Could you check a few things on this drawing? It's one solid part, dimensions in mm from its lowest x, y, z. Coordinates: 2 decimals unless noted, no trailing zeros. Order: outer loops, then holes, each group sorted by start corner. A loop starts at its lowest first (then second) coordinate and runs counter-clockwise, first axis right, second up.
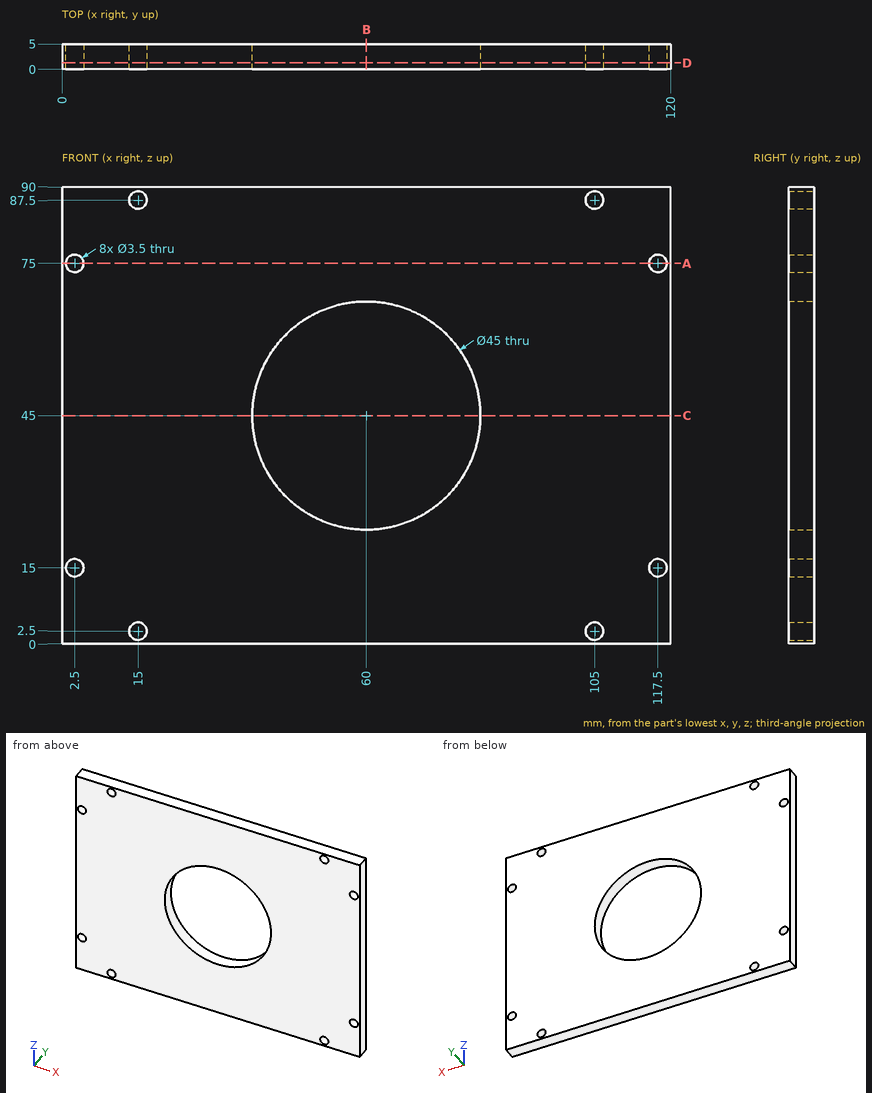
1. Imagine slicing it at A-A on z = 75. Please give me the cut outline in (x, y).
Completed:
outline: (0, 0) - (0.75, 0) - (0.75, 5) - (0, 5) - close; (4.25, 0) - (115.75, 0) - (115.75, 5) - (4.25, 5) - close; (119.25, 0) - (120, 0) - (120, 5) - (119.25, 5) - close
2. Please list where these lines run through material, in increasing order: probe 1 along X at (y, z) = (3.15, 2.5); probe 2 along Z at (x, y) = (105, 3.7); probe 3 along Z at (x, y) = (2.5, 2).
Completed:
probe 1: x = 0 to 13.25, 16.75 to 103.25, 106.75 to 120
probe 2: z = 0 to 0.75, 4.25 to 85.75, 89.25 to 90
probe 3: z = 0 to 13.25, 16.75 to 73.25, 76.75 to 90
3. Imagine slicing it at B-B on x = 60. Please give me the cut outline in (y, z).
Completed:
outline: (0, 0) - (5, 0) - (5, 22.5) - (0, 22.5) - close; (0, 67.5) - (5, 67.5) - (5, 90) - (0, 90) - close
4. Imagine slicing it at D-D on y = 1.3. Give the number of separate pieces and of enclosed holes in the cut face, then the cut area to 3 significant figures.
Completed:
separate pieces: 1
enclosed holes: 9
area: 9,130 mm2
5. Imagine slicing it at C-C on z = 45. Please give me the cut outline in (x, y).
Completed:
outline: (0, 0) - (37.5, 0) - (37.5, 5) - (0, 5) - close; (82.5, 0) - (120, 0) - (120, 5) - (82.5, 5) - close
